Model file for the job. Use its own axes, mm. Face numbers are marked on the shaded views. Give positions to 0.01 mm unless a question says otherwise; leave off trailing zeros. Order: outer loops, then holes, each group sorted by start corner. A loop starts at its lowest first (then second) coordinate and runs counter-clockwise, first axis right, second up. Notation, with made-up numbers: (76, -2.5) -> (97, -2.5) arc R30 cw to (97, 36.5) -> close; hole circle Ø6 at (-5, 24.5). An arc over 180 degrees is marked (long way). Answer in a Markdown table with one row per item. Add a question column.
Autodesk Inventor part; units mm, degrees
ref_plane "YZ Plane" through (0, 0, 0) normal (1, 0, 0) x (0, 1, 0)
ref_plane "XZ Plane" through (0, 0, 0) normal (0, 1, 0) x (-1, 0, 0)
ref_plane "XY Plane" through (0, 0, 0) normal (0, 0, 1) x (1, 0, 0)
ref_plane "Work Plane1" through (0, 0, 0) normal (0, 0, 1) x (1, 0, 0)
sketch "Sketch1" plane through (0, 0, 0) normal (0, 0, 1) x (1, 0, 0)
  circle A0 centre (0, -23.8125) radius 2.1526 construction
  circle A1 centre (20.6222, 11.9063) radius 2.1526 construction
  circle A2 centre (-20.6222, 11.9062) radius 2.1526 construction
  line L0 (2.7178, 3.2258) -> (-2.7178, 3.2258)
  line L1 (-3.2258, 2.7178) -> (-3.2258, -2.7178)
  line L2 (-2.7178, -3.2258) -> (2.7178, -3.2258)
  line L3 (3.2258, -2.7178) -> (3.2258, 2.7178)
  line L4 (3.2258, 3.2258) -> (-3.2258, -3.2258) construction
  line L5 (-3.2258, 3.2258) -> (3.2258, -3.2258) construction
  arc A3 (2.7178, -3.2258) -> (3.2258, -2.7178) centre (2.7178, -2.7178) ccw
  arc A4 (-3.2258, -2.7178) -> (-2.7178, -3.2258) centre (-2.7178, -2.7178) ccw
  arc A5 (-2.7178, 3.2258) -> (-3.2258, 2.7178) centre (-2.7178, 2.7178) ccw
  arc A6 (3.2258, 2.7178) -> (2.7178, 3.2258) centre (2.7178, 2.7178) ccw
  circle A7 centre (0, 0) radius 11.1125
  circle A8 centre (0, -23.8125) radius 4.7625
  circle A9 centre (-20.6222, 11.9062) radius 4.7625
  circle A10 centre (20.6222, 11.9063) radius 4.7625
  arc A11 (22.9921, 7.7752) -> (4.7625, -23.7993) centre (41.0481, -23.6991) ccw
  arc A12 (-18.2296, 16.0241) -> (18.2296, 16.0241) centre (0, 47.3982) ccw
  arc A13 (-4.7625, -23.7993) -> (-22.9921, 7.7752) centre (-41.0481, -23.6991) ccw
  circle A14 centre (0, -23.8125) radius 2.2479
  circle A15 centre (20.6222, 11.9062) radius 2.2479
  circle A16 centre (-20.6222, 11.9063) radius 2.2479
  point P0 (18.2296, 16.0241)
  point P1 (-18.2296, 16.0241)
  point P2 (-22.9921, 7.7752)
  point P3 (-4.7625, -23.7993)
  dimension "d3" = 9.525
  dimension "d0" = 0.508
  dimension "d1" = 6.4516
  dimension "d2" = 22.225
  dimension "d6" = 360
  dimension "d8" = 4.4958
  dimension "d11" = 360
extrude "Extrusion1" add sketch "Sketch1" along normal blind 1.5
properties part number "3in flex wheel holder"
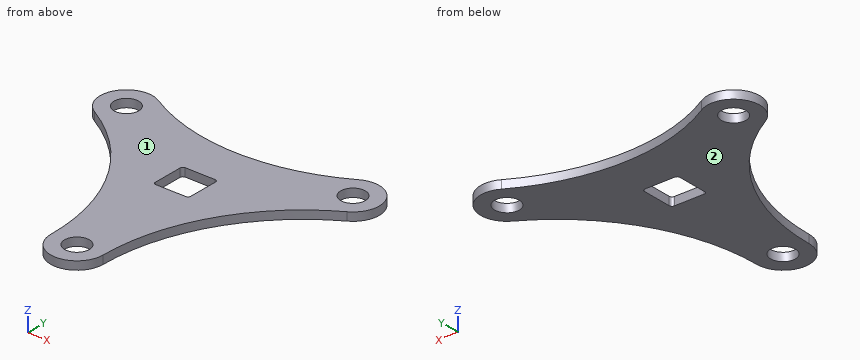
Item 1: Saw through at B-B on x = 21. List the corners of the cut face in (y, z), plus the area to 3 significant figures.
Item 2: Saw through at D-D on y = 13. List the corners of the cut face in (x, z).
Item 3: Wall check: line 1 (Y direction, x = 0, z = 0.4) (1 decimal); line 2 (X direction, y = -24, z = 1.45); line 3 (Y direction, x = 1.5, z = 0.8). Give the ranges that are in metal, low to high.
Item 4: Saw through at C-C on z = 0.7. List the corners of the cut face in (x, y) (1 decimal).
Item 5: Pin check, flat tips, straight feed: pin 1 Ø6 at (x, y) = (20.62, 11.91) entering from -Z; pin 2 Ø0.8 at (x, z) = (-1, 0.5) entering from +Y; pin 3 Ø2.5 at (x, y) = (-20.62, 11.91) entering from -Z. Stop position of each tip, or through.
Item 6: Two-plate mould, pull along Z, no slides. Class the marked faces 1 and 2: pulls with the +Z half, pulls with the -Z half, needs draft (parallel to the pull), parting line crosses it, or undercut.
Item 7: Saw through at A-A on x = 0. List the corners of the cut face in (y, z) (1 decimal), plus the area to 3 significant figures.
Evaluation:
| question | item | result |
|---|---|---|
| 1 | outline | (6.55, 0) -> (9.69, 0) -> (9.69, 1.5) -> (6.55, 1.5) -> close; (14.12, 0) -> (16.65, 0) -> (16.65, 1.5) -> (14.12, 1.5) -> close |
| 1 | area | 8.51 mm2 |
| 2 | outline | (-25.26, 0) -> (-22.59, 0) -> (-22.59, 1.5) -> (-25.26, 1.5) -> close; (-18.66, 0) -> (-11.55, 0) -> (-11.55, 1.5) -> (-18.66, 1.5) -> close; (11.55, 0) -> (18.66, 0) -> (18.66, 1.5) -> (11.55, 1.5) -> close; (22.59, 0) -> (25.26, 0) -> (25.26, 1.5) -> (22.59, 1.5) -> close |
| 3 | line 1 | y = -28.6 to -26.1, -21.6 to -3.2, 3.2 to 11.1 |
| 3 | line 2 | x = -4.76 to -2.24, 2.24 to 4.76 |
| 3 | line 3 | y = -28.33 to -25.49, -22.14 to -3.23, 3.23 to 11.14 |
| 4 | outline | (-23, 7.8) arc R36.3 cw to (-4.8, -23.8) arc R4.8 ccw to (4.8, -23.8) arc R36.3 cw to (23, 7.8) arc R4.8 ccw to (18.2, 16) arc R36.3 cw to (-18.2, 16) arc R4.8 ccw to start; hole circle Ø4.5 at (-20.6, 11.9); hole (-3.2, -2.7) arc R0.5 ccw to (-2.7, -3.2) -> (2.7, -3.2) arc R0.5 ccw to (3.2, -2.7) -> (3.2, 2.7) arc R0.5 ccw to (2.7, 3.2) -> (-2.7, 3.2) arc R0.5 ccw to (-3.2, 2.7) -> close; hole circle Ø4.5 at (0, -23.8); hole circle Ø4.5 at (20.6, 11.9) |
| 5 | pin 1 | stops at z = 0 |
| 5 | pin 2 | stops at y = 11.14 |
| 5 | pin 3 | passes through |
| 6 | face 1 | pulls with the +Z half |
| 6 | face 2 | pulls with the -Z half |
| 7 | outline | (-28.6, 0) -> (-26.1, 0) -> (-26.1, 1.5) -> (-28.6, 1.5) -> close; (-21.6, 0) -> (-3.2, 0) -> (-3.2, 1.5) -> (-21.6, 1.5) -> close; (3.2, 0) -> (11.1, 0) -> (11.1, 1.5) -> (3.2, 1.5) -> close |
| 7 | area | 43.1 mm2 |
